Verification items for this drawing (mm, ordinates from the low corner). Coordinates: 2 decimals unless noted, no trailing zeros. Write each loop counter-clockwise with the first axis right and the second up, starting at its lowest first coordinate (ties: lowest second). Pieces come first, ordered by that corner, then holes. Notation, with made-up numbers: M 2,-10.75 L 20,-10.75 A18 ccw 20,-0.75 Z; hole C -1,20.25 d5. An arc over 180 degrees is marked long. Put each result on its own line as item: value. Start each with the question number.
1) Cross-section at B-B on x = 6. Record the cut outline in (y, z), plus the area to 3 significant figures.
2) Cross-section at A-A on z = 2.5. Record the cut outline in (x, y), plus the area to 3 significant figures.
3) Scan lines: line 1 along Y through (x, z) = (32.5, 1.8); line 2 along Y through (x, z) = (43.5, 2.5); line 3 along X through (y, z) = (38, 3.75). Record each from-to range of solid material in increasing order.
4) Mould release check, pull along X, two halves, no side actions. Record for the marked faces 1, 2 and 3: released by +X, released by -X, zero draft, split by the parting line, or undercut.
5) Gauge pin test, flat end, axial feed: pin 1 (1 mm diameter, centred on x = 54, y = 28.5, fed in from +Z). Record the tip position at first contact, or that the pin passes through.
6) Cross-section at C-C on y = 32.5. Record the cut outline in (x, z).
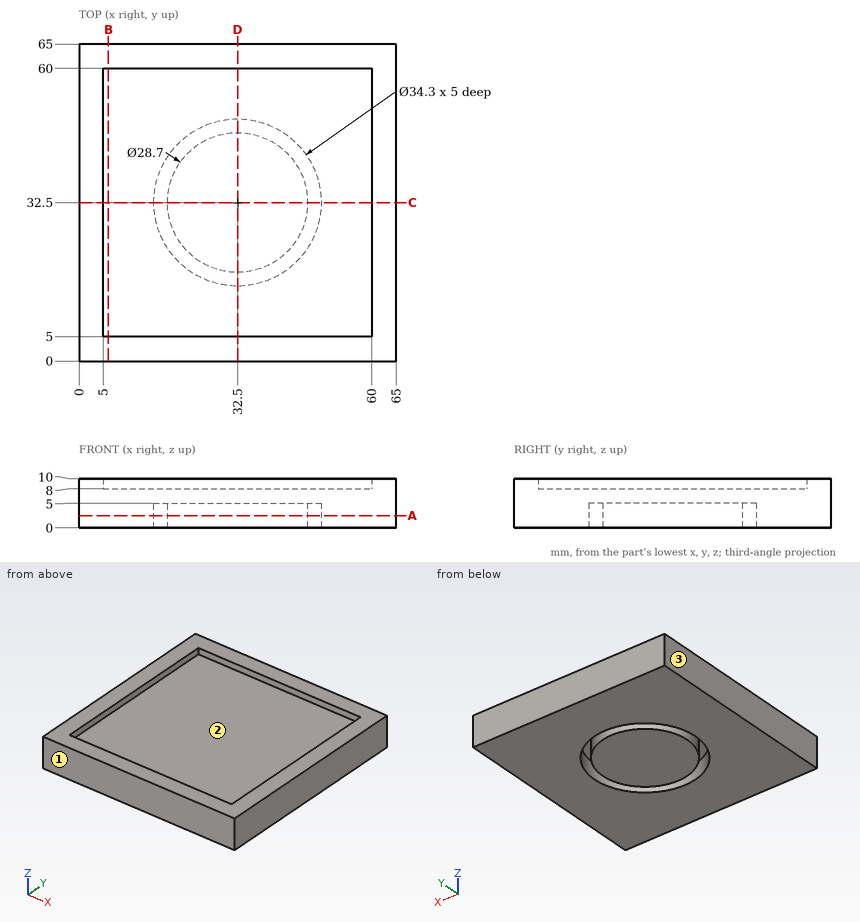
Answer key:
1. outline: M 0,0 L 65,0 L 65,10 L 60,10 L 60,8 L 5,8 L 5,10 L 0,10 Z
1. area: 540 mm²
2. outline: M 0,0 L 65,0 L 65,65 L 0,65 Z; C 32.5,32.5 d28.7; hole C 32.5,32.5 d34.3
2. area: 3,950 mm²
3. line 1: y = 0 to 15.35, 18.15 to 46.85, 49.65 to 65
3. line 2: y = 0 to 19.34, 23.28 to 41.72, 45.66 to 65
3. line 3: x = 0 to 16.26, 19.25 to 45.75, 48.74 to 65
4. face 1: zero draft
4. face 2: undercut
4. face 3: released by -X
5. pin 1: stops at z = 8
6. outline: M 0,0 L 15.35,0 L 15.35,5 L 18.15,5 L 18.15,0 L 46.85,0 L 46.85,5 L 49.65,5 L 49.65,0 L 65,0 L 65,10 L 60,10 L 60,8 L 5,8 L 5,10 L 0,10 Z
